```python
from build123d import *

# Parameters (mm, degrees)
CROQUIS1_R              = 2.5
SALIENTE_EXTRUIR1_DEPTH = 8
CROQUIS2_R              = 5
SALIENTE_EXTRUIR2_DEPTH = 3
CROQUIS3_W              = 1.4
CROQUIS3_H              = 11
CORTAR_EXTRUIR2_DEPTH   = 2.5
CORTAR_EXTRUIR2_TAPER   = 9


with BuildPart() as part:
    # Croquis1 → Saliente-Extruir1 (new body)
    with BuildSketch(Plane.XY):
        Circle(CROQUIS1_R)
    extrude(amount=SALIENTE_EXTRUIR1_DEPTH)

    # Croquis2 → Saliente-Extruir2 (add)
    with BuildSketch(Plane.XY):
        Circle(CROQUIS2_R)
    extrude(amount=-SALIENTE_EXTRUIR2_DEPTH)

    # Croquis3 → Cortar-Extruir2 (cut)
    with BuildSketch(Plane(origin=(0, 0, -3), x_dir=(-1, 0, 0), z_dir=(0, 0, -1))):
        Rectangle(CROQUIS3_W, CROQUIS3_H)
    extrude(amount=-CORTAR_EXTRUIR2_DEPTH, taper=CORTAR_EXTRUIR2_TAPER, mode=Mode.SUBTRACT)


solid = part.part
```
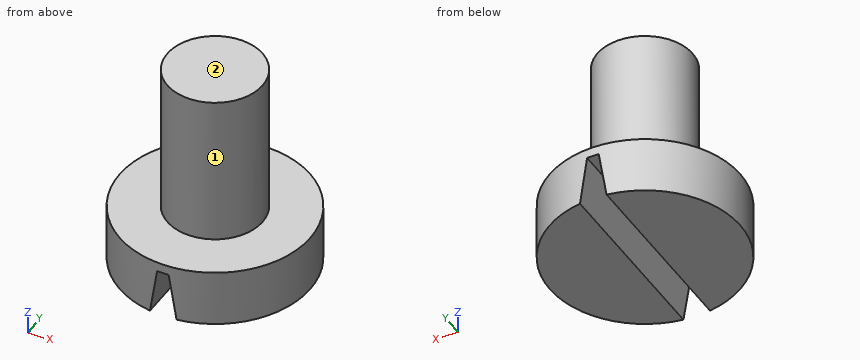
Part model, mm, in its own coordinate system. Face numbers are marked on the shaded views. A direction names the side the tool comes from. Round coordinates to 2 decimals unless told otherwise and drop trailing zeros. Write each loop counter-clockwise with the first axis right and the second up, starting at its lowest first coordinate (ties: lowest second). Pieces come first, ordered by that corner, then holes. Notation, with made-up numbers: (73.5, -1.5) -> (115.5, -1.5) arc R26 cw to (115.5, 14.5) -> close; hole circle Ø5 at (23, -1). An arc over 180 degrees is marked (long way). Return JSON: item names as keys, results as strings. Group by question number.
Q1. Saw through at B-B on z = 3. Write the cut outline in (x, y), plus the area to 3 significant figures.
Q2. Probe L1, parallel to Z at x = 1.25, y = -2.25; L2, parallel to Z at x = 0, y = 3.25; L3, parallel to X at y = 4, z = -2.25. List the from-to ranges inside material, lowest first. Write a range as [from, to].
Q3. Pin check, flat tips, straight feed: pin 1 (4 mm diameter, centred on x = -2.5, z = 5.5, fed in from +Y); pin 2 (2 mm diameter, centred on x = -3.5, z = -1.5, fed in from -Y); pin 3 (2 mm diameter, centred on y = -0.5, z = 3.5, fed in from -X). Stop position of each tip, or through.
Q4. Saw through at C-C on x = -1.25. Write the cut outline in (y, z).
Q5. Saw through at A-A on x = 0. Write the cut outline in (y, z), plus the area to 3 significant figures.
Q6. Saw through at D-D on x = 3.75. Write the cut outline in (y, z), plus the area to 3 significant figures.
Q7. Which spindle directions (+Z, -Z, +X, -X, +Y, -Y) get a long thin tool onto all of the face, cutting with end or side? Do the marked faces 1 and 2. Say none if no direction does.
Answer:
{
 "1": {"outline": "circle Ø5 at (0, 0)", "area": "19.6 mm2"},
 "2": {"L1": "[-3, 0]", "L2": "[-0.5, 0]", "L3": "[-3, -0.58], [0.58, 3]"},
 "3": {"pin 1": "y = 2.45", "pin 2": "y = -4.33", "pin 3": "x = -2.5"},
 "4": {"outline": "(-4.84, -3) -> (4.84, -3) -> (4.84, 0) -> (2.17, 0) -> (2.17, 8) -> (-2.17, 8) -> (-2.17, 0) -> (-4.84, 0) -> close"},
 "5": {"outline": "(-5, -0.5) -> (5, -0.5) -> (5, 0) -> (2.5, 0) -> (2.5, 8) -> (-2.5, 8) -> (-2.5, 0) -> (-5, 0) -> close", "area": "45.0 mm2"},
 "6": {"outline": "(-3.31, -3) -> (3.31, -3) -> (3.31, 0) -> (-3.31, 0) -> close", "area": "19.8 mm2"},
 "7": {"face 1": "+Z", "face 2": "+Z, +X, -X, +Y, -Y"}
}
